For this review, take the finished solid that the model builds, in its own axes (mm). A direction names the side the tool comes from. Coordinates: 2 decimals unless noted, no trailing zeros. Order: outer loops, then holes, each group sorted by start corner. A loop starts at its lowest first (then second) coordinate and runs counter-clockwise, first axis right, second up. Notation, with made-up numbers: (-11.75, 71.25) -> (2.25, 71.25) arc R23 cw to (2.25, 98.25) -> close; hole circle Ø10 at (-9, 69.25). An arc over 180 degrees is marked (long way). Write item = value, one per line. Start each with the question number.
1) Insertion check: pin 1 Ø1 at (y, z) = (-5, -1) entering from +X; pin 2 Ø0.6 at (y, z) = (-5.5, -2) entering from -X; pin 3 Ø1 at (x, z) = (-0.5, 1.5) entering from +Y. Each pin has a flat end and moves straight along its axis. Give the tip position at first contact, or say it passes through.
2) Consider section A-A on y = -3.25. Give the boundary of the cut face in (x, z).
3) Machinability: for faces 4 (the face through (0.191, -4, -2)), 5 (the face through (0.191, -4.4, 1.9)), 6 (the face through (0, -0.439, 1)), 7 (the face through (-1.27, -4.38, 0.03)), 8 (the face through (-0.191, -4, -2)), which of the approach directions +Z, -Z, +X, -X, +Y, -Y give a long, thin tool a straight path to every point of the face, cutting with its end or side? Answer none if there is none.
4) Draft analysis for pull direction Z (two halves, no side actions). For faces 1 (the face through (1.27, -4.38, -0.03)), 2 (the face through (-0.191, -4.4, 1.9)), 3 (the face through (0, -4.249, 1)), state which applies: +Z half, -Z half, draft (parallel to the pull), parting line (faces both ways), or undercut.
5) Wall thickness on probe 1 along Z at (x, y) = (0.15, -2.5); probe 2 along X at (y, z) = (-4.75, 1.4); probe 3 along X at (y, z) = (-0.25, 0.05): over which ranges is each line inside the solid? List them lowest first. Write a range as [from, to].
from build123d import *

# Parameters (mm, degrees)
F1_DEPTH = 8.89
F4_W     = 3.81
F4_H     = 1.27
F5_DEPTH = 12.7


with BuildPart() as f1:
    # F0 (on Front) → F1 (new body)
    with BuildSketch(Plane.XZ):
        with BuildLine():
            Line((0.1912181615, -2.54), (0.1912181615, -1.2555220487))
            ThreePointArc((0.1912181615, -1.2555220487), (1.27, 0), (0.1912181615, 1.2555220487))
            Line((0.1912181615, 1.2555220487), (0.1912181615, 2.54))
            Line((0.1912181615, 2.54), (-0.1912181615, 2.54))
            Line((-0.1912181615, 2.54), (-0.1912181615, 1.2555220487))
            ThreePointArc((-0.1912181615, 1.2555220487), (-1.27, 0), (-0.1912181615, -1.2555220487))
            Line((-0.1912181615, -1.2555220487), (-0.1912181615, -2.54))
            Line((-0.1912181615, -2.54), (0.1912181615, -2.54))
        make_face()
    extrude(amount=F1_DEPTH)

    # F2 (on Right) → F3 (revolve)
    with BuildSketch(Plane.YZ):
        with BuildLine():
            Line((0, 0), (0, -1.2554830802))
            ThreePointArc((0, -1.2554830802), (0.8877605997, -0.8877605997), (1.2554830802, 0))
            Line((1.2554830802, 0), (0, 0))
        make_face()
    revolve(axis=Axis((0, 0.6277415401, 0), (0, -1, 0)))

    # F4 (on face) → F5 (cut, symmetric)
    with BuildSketch(Plane.YZ.offset(0.1912181615)):
        with Locations((-2.3436378688, 1.2555220487)):
            Rectangle(F4_W, F4_H)
    extrude(amount=F5_DEPTH, both=True, mode=Mode.SUBTRACT)


solid = f1.part
Answer sheet:
q1.pin_1 = 1.17
q1.pin_2 = -0.19
q1.pin_3 = 0.64
q2.outline = (-1.11, 0.62) arc R1.27 ccw to (-0.19, -1.26) -> (-0.19, -2.54) -> (0.19, -2.54) -> (0.19, -1.26) arc R1.27 ccw to (1.11, 0.62) -> close; (-0.19, 1.89) -> (0.19, 1.89) -> (0.19, 2.54) -> (-0.19, 2.54) -> close
q3.face_4 = -Z, +X, +Y, -Y
q3.face_5 = +Z, +X, +Y, -Y
q3.face_6 = +X, -X
q3.face_7 = -X, +Y, -Y
q3.face_8 = -Z, -X, +Y, -Y
q4.face_1 = parting line
q4.face_2 = draft
q4.face_3 = undercut
q5.probe_1 = [-2.54, 0.62], [1.89, 2.54]
q5.probe_2 = [-0.19, 0.19]
q5.probe_3 = [-1.27, 1.27]
